Here's how the part is built. I have some questions about the finished solid (model axes, mm). Face numbers are marked on the shaded views. A direction names the side the tool comes from. Coordinates: 2 decimals unless noted, no trailing zeros. Write each loop counter-clockwise with the first axis right and the second up, starting at its lowest first coordinate (ties: lowest second). Pieces come first, ordered by that corner, then holes.
Item 1: Please list where these lines run through material, in increasing order: line 1 (Y direction, x = -38.45, z = -34); line 2 (Z direction, x = -39.35, y = -20); line 3 (X direction, y = -22, z = 23).
Item 2: For the marked faces 1 and 2, which set-ups out of +Z, -Z, +X, -X, +Y, -Y let a thin tool reach every point of the face, with its end or its side?
Item 3: I want a section at A-A (x = -18). Please give me the cut outline in (y, z).
Item 4: I want a section at B-B (y = -29). Please give me the cut outline in (x, z), and give its area (3 significant figures).
Item 5: If we mould it in two halves opening along X, with no side actions, what happens to the marked faces 3, 4 and 5? For each: pulls with the +X half, pulls with the -X half, needs draft (parallel to the pull), parting line crosses it, or undercut.
Item 6: I want a section at D-D (x = -32.5). Please give me the cut outline in (y, z), and give its area (3 significant figures).
Item 7: I want a section at C-C (z = -13.5). Please give me the cut outline in (x, y).
Item 8: I'm going to push a flat-ended pin straight in: P1, Ø4, axis at x = 14.5, z = 30.5, coming from the +Y side. Where does the tip first touch, or does it pass through?
from build123d import *

# Parameters (mm, degrees)
F0_W     = 81.5
F0_H     = 78
F0_W_2   = 75.5
F0_H_2   = 72
F1_DEPTH = 33
F2_W     = 81.5
F2_H     = 78
F2_W_2   = 56
F2_H_2   = 56
F3_DEPTH = 3
F4_R     = 0.75
F5_DEPTH = 111.5


with BuildPart() as f1:
    # F0 (on Front) → F1 (new body)
    with BuildSketch(Plane.XZ):
        Rectangle(F0_W, F0_H)
        Rectangle(F0_W_2, F0_H_2, mode=Mode.SUBTRACT)
    extrude(amount=F1_DEPTH)

    # F2 (on face) → F3 (join)
    with BuildSketch(Plane.XZ.offset(33)):
        Rectangle(F2_W, F2_H)
        Rectangle(F2_W_2, F2_H_2, mode=Mode.SUBTRACT)
    extrude(amount=-F3_DEPTH)

    # F4 (on face) → F5 (cut)
    with BuildSketch(Plane.YZ.offset(40.75)):
        with Locations((-10, -34)):
            Circle(F4_R)
        with Locations((-20, -34)):
            Circle(F4_R)
    extrude(amount=-F5_DEPTH, mode=Mode.SUBTRACT)


solid = f1.part
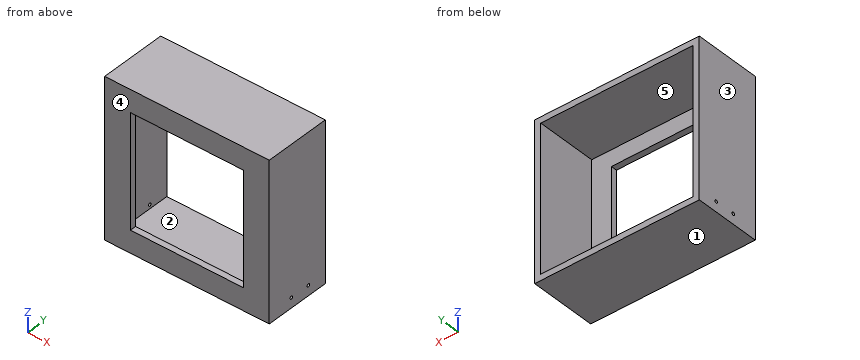
Answer:
1. line 1: y = -33 to -20.75, -19.25 to -10.75, -9.25 to 0
1. line 2: z = -39 to -34.75, -33.25 to 39
1. line 3: x = -40.75 to -37.75, 37.75 to 40.75
2. face 1: -Z, +X, -X, +Y, -Y
2. face 2: +Y
3. outline: (-33, -39) - (0, -39) - (0, -36) - (-30, -36) - (-30, -28) - (-33, -28) - close; (-33, 28) - (-30, 28) - (-30, 36) - (0, 36) - (0, 39) - (-33, 39) - close
4. outline: (-40.75, -39) - (40.75, -39) - (40.75, 39) - (-40.75, 39) - close; hole (-37.75, -36) - (37.75, -36) - (37.75, 36) - (-37.75, 36) - close
4. area: 921 mm2
5. face 3: pulls with the -X half
5. face 4: needs draft
5. face 5: undercut
6. outline: (-33, -39) - (0, -39) - (0, -36) - (-30, -36) - (-30, 36) - (0, 36) - (0, 39) - (-33, 39) - close
6. area: 414 mm2
7. outline: (-40.75, -33) - (-28, -33) - (-28, -30) - (-37.75, -30) - (-37.75, 0) - (-40.75, 0) - close; (28, -33) - (40.75, -33) - (40.75, 0) - (37.75, 0) - (37.75, -30) - (28, -30) - close
8. P1: stops at y = -30
